from build123d import *

# Parameters (mm, degrees)
SKETCH1_W                 = 279.4
SKETCH1_H                 = 76.2
BOSS_EXTRUDE1_DEPTH       = 3
SKETCH3_W                 = 3
SKETCH3_H                 = 15
SKETCH3_H_2               = 7.8
CUT_EXTRUDE1_DEPTH        = 145.833352512
LPATTERN1_COUNT           = 4
LPATTERN1_PITCH           = 22.8
MIRROR1_COPY_1_SKETCH_W   = 3
MIRROR1_COPY_1_SKETCH_H   = 15
MIRROR1_COPY_1_SKETCH_H_2 = 7.8
MIRROR1_COPY_1_DEPTH      = 145.833352512
MIRROR1_COPY_2_SKETCH_W   = 3
MIRROR1_COPY_2_SKETCH_H   = 15
MIRROR1_COPY_2_SKETCH_H_2 = 7.8
MIRROR1_COPY_2_DEPTH      = 145.833352512
MIRROR1_COPY_3_SKETCH_W   = 3
MIRROR1_COPY_3_SKETCH_H   = 15
MIRROR1_COPY_3_SKETCH_H_2 = 7.8
MIRROR1_COPY_3_DEPTH      = 145.833352512
SKETCH4_W                 = 3
SKETCH4_H                 = 15
CUT_EXTRUDE2_DEPTH        = 10
LPATTERN2_COUNT           = 3
LPATTERN2_PITCH           = 22.8
MIRROR2_COPY_1_SKETCH_W   = 3
MIRROR2_COPY_1_SKETCH_H   = 15
MIRROR2_COPY_1_DEPTH      = 10
MIRROR2_COPY_2_SKETCH_W   = 3
MIRROR2_COPY_2_SKETCH_H   = 15
MIRROR2_COPY_2_DEPTH      = 10
SKETCH5_W                 = 3
SKETCH5_H                 = 7.8
BOSS_EXTRUDE2_DEPTH       = 3
LPATTERN3_COUNT           = 8
LPATTERN3_PITCH           = 22.8


with BuildPart() as part:
    # Sketch1 → Boss-Extrude1 (new body)
    with BuildSketch(Plane(origin=(0, 0, 0), x_dir=(0, 0, -1), z_dir=(1, 0, 0))):
        Rectangle(SKETCH1_W, SKETCH1_H)
    extrude(amount=-BOSS_EXTRUDE1_DEPTH)

    # Sketch3 → Cut-Extrude1 (cut, through all)
    with BuildSketch(Plane.ZY.offset(3)):
        with Locations((-102.15, 22.8)):
            Rectangle(SKETCH3_W, SKETCH3_H)
        with Locations((-138.2, 34.2)):
            Rectangle(SKETCH3_W, SKETCH3_H_2)
    cut_extrude1 = extrude(amount=-CUT_EXTRUDE1_DEPTH, mode=Mode.SUBTRACT)

    # LPattern1: Cut-Extrude1 ×4
    with Locations(*[(0, -i * LPATTERN1_PITCH, 0) for i in range(1, LPATTERN1_COUNT)]):
        add(cut_extrude1, mode=Mode.SUBTRACT)

    # Mirror1: Cut-Extrude1 across plane
    add(cut_extrude1.mirror(Plane.XY), mode=Mode.SUBTRACT)

    # Mirror1 copy 1 sketch → Mirror1 copy 1 (cut, through all)
    with BuildSketch(Plane(origin=(-3, -22.8, 0), x_dir=(0, 0, -1), z_dir=(-1, 0, 0))):
        with Locations((-102.15, -22.8)):
            Rectangle(MIRROR1_COPY_1_SKETCH_W, MIRROR1_COPY_1_SKETCH_H)
        with Locations((-138.2, -34.2)):
            Rectangle(MIRROR1_COPY_1_SKETCH_W, MIRROR1_COPY_1_SKETCH_H_2)
    extrude(amount=-MIRROR1_COPY_1_DEPTH, mode=Mode.SUBTRACT)

    # Mirror1 copy 2 sketch → Mirror1 copy 2 (cut, through all)
    with BuildSketch(Plane(origin=(-3, -45.6, 0), x_dir=(0, 0, -1), z_dir=(-1, 0, 0))):
        with Locations((-102.15, -22.8)):
            Rectangle(MIRROR1_COPY_2_SKETCH_W, MIRROR1_COPY_2_SKETCH_H)
        with Locations((-138.2, -34.2)):
            Rectangle(MIRROR1_COPY_2_SKETCH_W, MIRROR1_COPY_2_SKETCH_H_2)
    extrude(amount=-MIRROR1_COPY_2_DEPTH, mode=Mode.SUBTRACT)

    # Mirror1 copy 3 sketch → Mirror1 copy 3 (cut, through all)
    with BuildSketch(Plane(origin=(-3, -68.4, 0), x_dir=(0, 0, -1), z_dir=(-1, 0, 0))):
        with Locations((-102.15, -22.8)):
            Rectangle(MIRROR1_COPY_3_SKETCH_W, MIRROR1_COPY_3_SKETCH_H)
        with Locations((-138.2, -34.2)):
            Rectangle(MIRROR1_COPY_3_SKETCH_W, MIRROR1_COPY_3_SKETCH_H_2)
    extrude(amount=-MIRROR1_COPY_3_DEPTH, mode=Mode.SUBTRACT)

    # Sketch4 → Cut-Extrude2 (cut)
    with BuildSketch(Plane(origin=(0, 0, 0), x_dir=(0, 0, -1), z_dir=(1, 0, 0))):
        with Locations((-89.15, 22.8)):
            Rectangle(SKETCH4_W, SKETCH4_H)
    cut_extrude2 = extrude(amount=-CUT_EXTRUDE2_DEPTH, mode=Mode.SUBTRACT)

    # LPattern2: Cut-Extrude2 ×3
    with Locations(*[(0, -i * LPATTERN2_PITCH, 0) for i in range(1, LPATTERN2_COUNT)]):
        add(cut_extrude2, mode=Mode.SUBTRACT)

    # Mirror2: Cut-Extrude2 across plane
    add(cut_extrude2.mirror(Plane.XY), mode=Mode.SUBTRACT)

    # Mirror2 copy 1 sketch → Mirror2 copy 1 (cut)
    with BuildSketch(Plane(origin=(0, -22.8, 0), x_dir=(0, 0, 1), z_dir=(1, 0, 0))):
        with Locations((-89.15, -22.8)):
            Rectangle(MIRROR2_COPY_1_SKETCH_W, MIRROR2_COPY_1_SKETCH_H)
    extrude(amount=-MIRROR2_COPY_1_DEPTH, mode=Mode.SUBTRACT)

    # Mirror2 copy 2 sketch → Mirror2 copy 2 (cut)
    with BuildSketch(Plane(origin=(0, -45.6, 0), x_dir=(0, 0, 1), z_dir=(1, 0, 0))):
        with Locations((-89.15, -22.8)):
            Rectangle(MIRROR2_COPY_2_SKETCH_W, MIRROR2_COPY_2_SKETCH_H)
    extrude(amount=-MIRROR2_COPY_2_DEPTH, mode=Mode.SUBTRACT)

    # Sketch5 → Boss-Extrude2 (add)
    with BuildSketch(Plane(origin=(0, 38.1, 0), x_dir=(1, 0, 0), z_dir=(0, 1, 0))):
        with Locations((-1.5, -79.8)):
            Rectangle(SKETCH5_W, SKETCH5_H)
    boss_extrude2 = extrude(amount=BOSS_EXTRUDE2_DEPTH)

    # LPattern3: Boss-Extrude2 ×8
    with Locations(*[(0, 0, -i * LPATTERN3_PITCH) for i in range(1, LPATTERN3_COUNT)]):
        add(boss_extrude2)


solid = part.part
Check sheet for the modelled part. Datum: model origin and axes. Units: mm. Coordinates: 2 decimals unless noted, no trailing zeros. Write each loop counter-clockwise with the first axis right and the second up, starting at its lowest first coordinate (ties: lowest second). Pieces come first, ordered by that corner, then holes.
Item 1: Cross-section at B-B on x = -2.3. Count the separate pieces of the cut face and the enclosed holes in it, then the cut area to 3 significant figures.
Numbers:
separate pieces: 1
enclosed holes: 12
area: 20,800 mm2
Item 2: Scan lines: probe 1 along Z at (x, y) = (-1.15, -0.5); probe 2 along Z at (x, y) = (-2.8, -11.5); probe 3 along Y at (x, z) = (-0.25, 40). Record each from-to range of solid material in increasing order.
Numbers:
probe 1: z = -139.7 to -103.65, -100.65 to -90.65, -87.65 to 87.65, 90.65 to 100.65, 103.65 to 139.7
probe 2: z = -136.7 to 136.7
probe 3: y = -38.1 to 38.1
Item 3: Cross-section at A-A on y = 3. Record the boundary of the cut face in (x, z).
Numbers:
outline: (-3, -139.7) - (0, -139.7) - (0, -103.65) - (-3, -103.65) - close; (-3, -100.65) - (0, -100.65) - (0, -90.65) - (-3, -90.65) - close; (-3, -87.65) - (0, -87.65) - (0, 87.65) - (-3, 87.65) - close; (-3, 90.65) - (0, 90.65) - (0, 100.65) - (-3, 100.65) - close; (-3, 103.65) - (0, 103.65) - (0, 139.7) - (-3, 139.7) - close
Item 4: Cross-section at C-C on z = -112. Record the boundary of the cut face in (x, y).
Numbers:
outline: (-3, -38.1) - (0, -38.1) - (0, 38.1) - (-3, 38.1) - close
Item 5: Depth check by flat-ended pin: pin 1 Ø1.5 at (x, y) = (-2, 10) entering from -Z. Enter the tip coordinate at first touch or a pass-through.
Numbers:
pin 1: stops at z = -136.7
